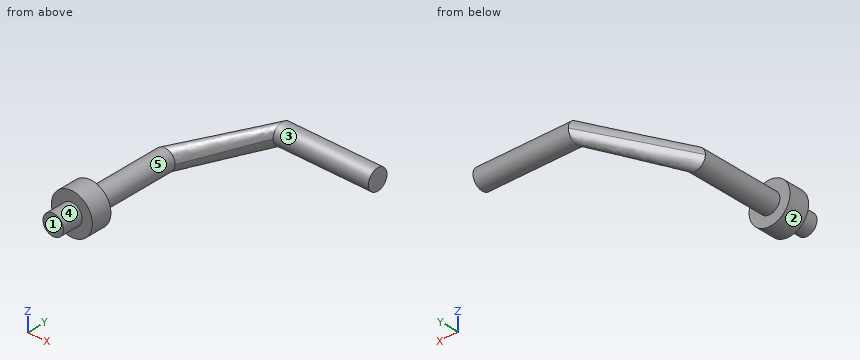
Autodesk Inventor part; units mm, degrees
ref_plane "Work Plane1" through (15, 0, 0) normal (1, 0, 0) x (0, 1, 0)
ref_plane "XZ Plane" through (0, 0, 0) normal (0, 1, 0) x (-1, 0, 0)
ref_plane "XY Plane" through (0, 0, 0) normal (0, 0, 1) x (1, 0, 0)
sketch "Sketch1" plane through (0, 0, 0) normal (0, 1, 0) x (-1, 0, 0)
  circle A0 centre (0, 0) radius 5
  dimension "d0" = 10
extrude "Extrusion1" add sketch "Sketch1" along normal blind 5
sketch "Sketch2" plane through (0, 0, 0) normal (0, -1, 0) x (1, 0, 0)
  circle A0 centre (0, 0) radius 2.5
  dimension "d3" = 5
extrude "Extrusion2" add sketch "Sketch2" along normal blind 5
sketch "Sketch3" plane through (0, 5, 0) normal (0, 1, 0) x (1, 0, 0)
  circle A0 centre (0, 0) radius 2.5
  dimension "d6" = 5
extrude "Extrusion3" add sketch "Sketch3" along normal blind 20
ref_plane "Work Plane1" through (15, 0, 0) normal (1, 0, 0) x (0, 1, 0)
sketch "Sketch6" plane through (15, 0, 0) normal (1, 0, 0) x (0, 1, 0)
  line L0 (25, -2.5) -> (25, 2.5)
  line L1 (25, 0) -> (40.064, 0)
  line L2 (40.064, 0) -> (40.064, 4.909)
  circle A0 centre (40.064, 4.909) radius 2.5
  point P0 (0, 0)
  dimension "d28" = 15.064
  dimension "d29" = 4.909
  dimension "d30" = 5
extrude "Extrusion6" add sketch "Sketch6" along normal blind 25
loft "Loft3" add section 1 edges at (-2.5, 25, 0) section 2 edges at (15, 37.564, 4.909)
sketch "Sketch7" plane through (40, 40.064, 4.909) normal (1, 0, 0) x (0, 0, -1)
  circle A0 centre (0, 0) radius 2.5
  point P0 (4.909, -40.064)
  dimension "d37" = 5
extrude "Extrusion7" cut sketch "Sketch7" against normal blind 1.733
properties part number "gud gear stand proto 1 2"
Design review of the part built by this model. Coordinates are the model's own, in mm. Face numbers are marked on the shaded views. A direction names the side the tool comes from. Give positions to 0.01 mm unless a question says otherwise; leave off trailing zeros. Order: outer loops, then holes, each group sorted by start corner. A loop starts at its lowest first (then second) coordinate and runs counter-clockwise, first axis right, second up. Notation, with made-up numbers: (65.25, 62) - (89.25, 62) arc R25 cw to (89.25, 99) - close; hole circle Ø8 at (43.25, -22). An arc over 180 degrees is marked (long way). Use a Markdown table: item, result. Add a question column.
(1) Add section A-A on y = 2. Give the boundary of the cut face in (x, z), then the cut area to 3 significant figures.
(2) Clearance check with flat-ended pins moving along their axes: P1, Ø1.5, axis at x = 3.5, z = 5.5, coming from the -Y side; P2, Ø1, axis at y = 29.5, z = 0, coming from the +X side; P3, Ø3, axis at x = 1.5, z = 0.5, coming from the +Y side. State where each tip first meets the part, or that it passes through.
(3) Mouldability with a two-part tool opening along Y and no side actions: class the marked faces 3, 4 and 5 as +Y half, -Y half, draft (parallel to the pull), parting line (faces both ways), or undercut.
(4) Add section B-B on x = 17.5. Give the boundary of the cut face in (y, z), then the cut area to 3 significant figures.
(5) Machinability: for the marked faces 1 and 2, which of the approach directions +Z, -Z, +X, -X, +Y, -Y give a long, thin tool a straight path to every point of the face, cutting with its end or side? Answer none if there is none.
(6) Wall thickness on probe 1 along Y at (x, z) = (-3, 1.25); probe 2 along Y at (x, z) = (4.5, 1); probe 3 along X at (y, z) = (25, -1): over which ranges is each line inside the solid? List them lowest first. Write a range as [from, to].
Report:
| question | item | result |
|---|---|---|
| 1 | outline | circle Ø10 at (0, 0) |
| 1 | area | 78.5 mm² |
| 2 | P1 | passes through |
| 2 | P2 | stops at x = 6.85 |
| 2 | P3 | stops at y = 30.39 |
| 3 | face 3 | parting line |
| 3 | face 4 | draft |
| 3 | face 5 | undercut |
| 4 | outline | circle Ø5 at (40.06, 4.91) |
| 4 | area | 19.6 mm² |
| 5 | face 1 | +Z, -Z, +X, -X, -Y |
| 5 | face 2 | -Y |
| 6 | probe 1 | y = [0, 5] |
| 6 | probe 2 | y = [0, 5], [27.02, 31.84] |
| 6 | probe 3 | x = [-2.29, 2.29] |
